```python
from build123d import *

# Parameters (mm, degrees)
F0_W     = 400
F0_H     = 100
F1_DEPTH = 100
F3_DEPTH = 20
F4_W     = 100
F4_H     = 50
F5_DEPTH = 50


with BuildPart() as f1:
    # F0 (on Top) → F1 (new body)
    with BuildSketch(Plane.XY):
        with Locations((70.573999, 8.728447)):
            Rectangle(F0_W, F0_H)
    extrude(amount=F1_DEPTH)

    # F2 (on face) → F3 (join)
    with BuildSketch(Plane.XY.offset(100)):
        Polygon((270.573999, -16.271553), (270.573999, 33.728447), (-129.426001, 28.728447), (-129.426001, -11.271553), align=None)
    extrude(amount=F3_DEPTH)

    # F4 (on face) → F5 (cut)
    with BuildSketch(Plane(origin=(-129.426001, 0, 0), x_dir=(0, -1, 0), z_dir=(-1, 0, 0))):
        with Locations((-8.728447, 50)):
            Rectangle(F4_W, F4_H)
    extrude(amount=-F5_DEPTH, mode=Mode.SUBTRACT)


solid = f1.part
```
CAD build for the part. Positions are in the model's coordinates, mm. A direction names the side the tool comes from. Coordinates: 2 decimals unless noted, no trailing zeros. Order: outer loops, then holes, each group sorted by start corner. A loop starts at its lowest first (then second) coordinate and runs counter-clockwise, first axis right, second up. Notation, with made-up numbers: (0, 4.5) - (23, 4.5) arc R28 ccw to (23, 42.5) - close; hole circle Ø5 at (60.5, -34.5). An arc over 180 degrees is marked (long way). Answer in a Markdown table with one row per item.
1. Drill centre lines: L1, parallel to Z at x = -104, y = 2.5; L2, parallel to Z at x = -97, y = -25.5; L3, parallel to Z at x = 16, y = 40. Where is each one in solid material? Low to high. Write a range as from..to.
Answer:
| item | result |
|---|---|
| L1 | 0..25, 75..120 |
| L2 | 0..25, 75..100 |
| L3 | 0..100 |
2. 3-axis set-ups, long thin cutter, end or side, ignore diameter. For faces 1 (the face through (-79.426, 9, 50)), 2 (the face through (270.574, 8, 59)), 3 (the face through (68, -26, 100)): which of +Z, -Z, +X, -X, +Y, -Y reach the whole face in a straight line?
Answer:
| item | result |
|---|---|
| face 1 | -X, +Y, -Y |
| face 2 | +Z, -Z, +X, +Y, -Y |
| face 3 | +Z, -X, -Y |
3. Slice it at B-B, the plane x = 86. List the corners of the cut face in (y, z), then the cut area to 3 significant figures.
Answer:
| item | result |
|---|---|
| outline | (-41.27, 0) - (58.73, 0) - (58.73, 100) - (31.42, 100) - (31.42, 120) - (-13.96, 120) - (-13.96, 100) - (-41.27, 100) - close |
| area | 10,900 mm² |
4. Slice it at D-D, the plane z = 108. List the corners of the cut face in (x, y).
Answer:
| item | result |
|---|---|
| outline | (-129.43, -11.27) - (270.57, -16.27) - (270.57, 33.73) - (-129.43, 28.73) - close |
5. Pull direction Z, two halves, no side cores. Call faces 4 (the face through (68, 9, 0)), 5 (the face through (68, 9, 120)), 6 (the face through (68, 58.728, 49)), 7 (the face through (-105, 9, 25)): +Z half, -Z half, draft (parallel to the pull), parting line (faces both ways), or undercut.
Answer:
| item | result |
|---|---|
| face 4 | -Z half |
| face 5 | +Z half |
| face 6 | draft |
| face 7 | undercut |
6. Slice it at C-C, the plane z = 62.5. List the corners of the cut face in (x, y).
Answer:
| item | result |
|---|---|
| outline | (-79.43, -41.27) - (270.57, -41.27) - (270.57, 58.73) - (-79.43, 58.73) - close |
7. Flat gauge pin, fed straight in: P1, Ø15, axis at x = -22.5, y = 45, coming from the +Z side. Where does the tip first touch, or does it go through?
Answer:
| item | result |
|---|---|
| P1 | z = 100 |
8. Slice it at A-A, the plane y = -7.5. List the corners of the cut face in (x, z).
Answer:
| item | result |
|---|---|
| outline | (-129.43, 0) - (270.57, 0) - (270.57, 120) - (-129.43, 120) - (-129.43, 75) - (-79.43, 75) - (-79.43, 25) - (-129.43, 25) - close |
